```python
from build123d import *

# Parameters (mm, degrees)
F1_DEPTH = 5
F0_W     = 75
F0_H     = 5
F2_DEPTH = 77
F3_SIZE  = 45
F4_SIZE  = 45
F5_R     = 3
F6_R     = 8
F8_D     = 10
F9_D     = 10


with BuildPart() as f1:
    # F0 (on Top) → F1 (new body)
    with BuildSketch(Plane.XY):
        Polygon((30, 23.6378825456), (55, 23.6378825456), (55, 124.6378825456), (0, 124.6378825456), (-75, 124.6378825456), (-75, 79.1378825456), (-75, 23.6378825456), (0, 23.6378825456), align=None)
        with BuildLine():
            ThreePointArc((36, 52.6378825456), (34.2426406871, 48.3952418585), (30, 46.6378825456))
            ThreePointArc((30, 46.6378825456), (24, 52.6378825456), (30, 58.6378825456))
            ThreePointArc((30, 58.6378825456), (34.2426406871, 56.8805232327), (36, 52.6378825456))
        make_face(mode=Mode.SUBTRACT)
        with BuildLine():
            ThreePointArc((-44, 79.1378825456), (-50, 73.1378825456), (-56, 79.1378825456))
            ThreePointArc((-56, 79.1378825456), (-50, 85.1378825456), (-44, 79.1378825456))
        make_face(mode=Mode.SUBTRACT)
        with BuildLine():
            ThreePointArc((36, 95.6378825456), (34.2426406871, 91.3952418585), (30, 89.6378825456))
            ThreePointArc((30, 89.6378825456), (25.7573593129, 99.8805232327), (36, 95.6378825456))
        make_face(mode=Mode.SUBTRACT)
    extrude(amount=F1_DEPTH)

    # F0 (on Top) → F2 (join)
    with BuildSketch(Plane.XY):
        with Locations((-37.5, 127.1378825456)):
            Rectangle(F0_W, F0_H)
        with Locations((-37.5, 21.1378825456)):
            Rectangle(F0_W, F0_H)
    extrude(amount=F2_DEPTH)

    # F3
    f3_edges = [f1.edges().sort_by_distance(p)[0] for p in [
        (0, 127.137883, 77),
    ]]
    chamfer(f3_edges, length=F3_SIZE)

    # F4
    f4_edges = [f1.edges().sort_by_distance(p)[0] for p in [
        (0, 21.137883, 77),
    ]]
    chamfer(f4_edges, length=F4_SIZE)

    # F5
    f5_edges = [f1.edges().sort_by_distance(p)[0] for p in [
        (-37.5, 124.637883, 5),
        (-37.5, 23.637883, 5),
    ]]
    fillet(f5_edges, radius=F5_R)

    # F6
    f6_edges = [f1.edges().sort_by_distance(p)[0] for p in [
        (-37.5, 18.637883, 0),
        (-37.5, 129.637883, 0),
    ]]
    fillet(f6_edges, radius=F6_R)

    # F8 (through all)
    with Locations(Plane.XZ.offset(-18.6378825456)):
        with Locations((-50, 37)):
            Hole(F8_D / 2)

    # F9 (through all)
    with Locations(Plane.XZ.offset(-18.6378825456)):
        with Locations((-50, 62)):
            Hole(F9_D / 2)


solid = f1.part
```
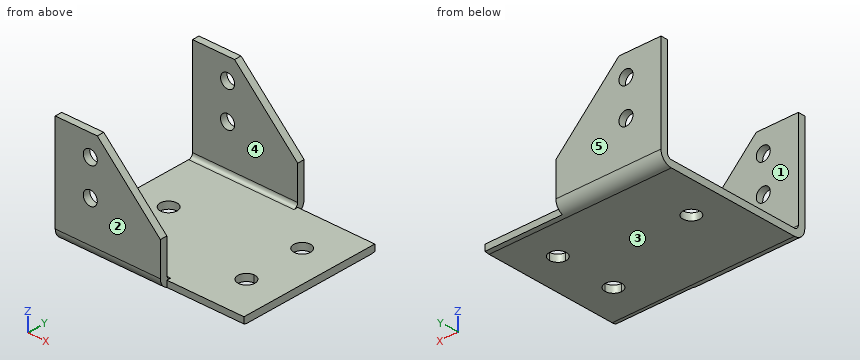
Can you work these out from the model? Positions are in its coordinate system, mm. Face numbers are marked on the shaded views. A direction names the side the tool comes from. Coordinates: 2 decimals unless noted, no trailing zeros. Order: outer loops, then holes, each group sorted by start corner. A loop starts at its lowest first (then second) coordinate and runs counter-clockwise, first axis right, second up. Notation, with made-up numbers: (37, 61.5) -> (78, 61.5) arc R21 cw to (78, 91.5) -> close; hole circle Ø11 at (82, -18). An arc over 180 degrees is marked (long way). Write each question's results on one line, items separated by ' | '.
Item 1: I want a section at A-A, the plane z = 37. Write out the boundary of the cut face in (x, y), then the cut area to 3 significant figures.
Results are:
outline: (-75, 18.64) -> (-55, 18.64) -> (-55, 23.64) -> (-75, 23.64) -> close; (-75, 124.64) -> (-55, 124.64) -> (-55, 129.64) -> (-75, 129.64) -> close; (-45, 18.64) -> (-5, 18.64) -> (-5, 23.64) -> (-45, 23.64) -> close; (-45, 124.64) -> (-5, 124.64) -> (-5, 129.64) -> (-45, 129.64) -> close | area: 600 mm²
Item 2: I want a section at C-C, the plane z = 48.5. Write out the boundary of the cut face in (x, y), then the cut area to 3 significant figures.
Results are:
outline: (-75, 18.64) -> (-16.5, 18.64) -> (-16.5, 23.64) -> (-75, 23.64) -> close; (-75, 124.64) -> (-16.5, 124.64) -> (-16.5, 129.64) -> (-75, 129.64) -> close | area: 585 mm²
Item 3: I want a section at B-B, the plane x = -50. Count the separate pieces of the cut face and the enclosed holes in it, then the cut area to 3 significant figures.
Results are:
separate pieces: 6 | enclosed holes: 0 | area: 991 mm²
Item 4: I want a section at D-D, the plane x = -15.5. Write out the boundary of the cut face in (y, z), then the cut area to 3 significant figures.
Results are:
outline: (18.64, 8) arc R8 ccw to (26.64, 0) -> (121.64, 0) arc R8 ccw to (129.64, 8) -> (129.64, 47.5) -> (124.64, 47.5) -> (124.64, 8) arc R3 cw to (121.64, 5) -> (26.64, 5) arc R3 cw to (23.64, 8) -> (23.64, 47.5) -> (18.64, 47.5) -> close | area: 956 mm²
Item 5: Which directions (+Z, -Z, +X, -X, +Y, -Y) give clear straight access to the entire face, cutting with the end or side of a thin tool? Please do the marked faces 1 and 2.
Results are:
face 1: +Z, +X, -X | face 2: +Z, -Z, +X, -X, -Y
Item 6: If we mould it in two halves opening along Y, with no side actions, what happens to the marked faces 3, 4 and 5? For each: +Y half, -Y half, draft (parallel to the pull), parting line (faces both ways), or undercut.
Results are:
face 3: draft | face 4: undercut | face 5: +Y half
Item 7: If I drill on line 1 along Y through (x, z) = (-39, 69.5); line 2 along Z through (x, y) = (-50, 127.35); line 3 along Z through (x, y) = (-50, 20.6), over which ranges is the centre line in solid material (lowest first)?
Results are:
line 1: 18.64 to 23.64, 124.64 to 129.64 | line 2: 2.4 to 32, 42 to 57, 67 to 77 | line 3: 2.75 to 32, 42 to 57, 67 to 77
Item 8: I'm going to push flat-ended pins straight in: pin 1 Ø6 at (x, y) = (-39.5, 96.5) entering from +Z; pin 2 Ø5 at (x, z) = (34.5, 3) entering from +Y; pin 3 Ø3.5 at (x, z) = (38.5, 3.5) entering from -Y. Where does each tip first touch, or does it pass through?
Results are:
pin 1: z = 5 | pin 2: y = 124.64 | pin 3: y = 23.64
